from build123d import *

# Parameters (mm, degrees)
SKETCH1_R           = 11.8
SKETCH1_R_2         = 1.4
BOSS_EXTRUDE2_DEPTH = 10


with BuildPart() as part:
    # Sketch1 → Boss-Extrude2 (new body)
    with BuildSketch(Plane(origin=(0, 0, 0), x_dir=(1, 0, 0), z_dir=(0, 1, 0))):
        Polygon((-12.5, 10.5), (-10.5, 12.5), (10.5, 12.5), (12.5, 10.5), (12.5, -10.5), (10.5, -12.5), (-10.5, -12.5), (-12.5, -10.5), align=None)
        with Locations(Location((0, 0, 0), (0, 0, 270))):
            Circle(SKETCH1_R, mode=Mode.SUBTRACT)
        with Locations(Location((-10, 10, 0), (0, 0, 270))):
            Circle(SKETCH1_R_2, mode=Mode.SUBTRACT)
        with Locations(Location((10, 10, 0), (0, 0, 270))):
            Circle(SKETCH1_R_2, mode=Mode.SUBTRACT)
        with Locations(Location((10, -10, 0), (0, 0, 270))):
            Circle(SKETCH1_R_2, mode=Mode.SUBTRACT)
        with Locations(Location((-10, -10, 0), (0, 0, 270))):
            Circle(SKETCH1_R_2, mode=Mode.SUBTRACT)
    extrude(amount=BOSS_EXTRUDE2_DEPTH)


solid = part.part
Can you work these out from the model? Positions are in its coordinate system, mm. Coordinates: 2 decimals unless noted, no trailing zeros. Write each loop counter-clockwise with the first axis right and the second up, starting at its lowest first coordinate (ties: lowest second). Pieces come first, ordered by that corner, then holes. Notation, with made-up numbers: (83, 25) -> (123, 25) arc R20 cw to (123, 42) -> close; hole circle Ø10 at (73.5, -16.5). An arc over 180 degrees is marked (long way). Write each question's results on one line, items separated by ' | '. Start each with the question number.
Q1. We'd pull the mould along X, two halves only. Please class faces 1 (the face through (10.95, 4.93, 8.97)), 2 (the face through (-12.5, 5, 0)), 3 (the face through (12, 5, 11)), 4 (the face through (10.95, 4.93, -11.03)): +X half, -X half, draft (parallel to the pull), parting line (faces both ways), or undercut.
Q2. Imagine slicing it at B-B (z = 0). Write out the boundary of the cut face in (x, y).
Q3. If I drill on probe 1 along X at (y, z) = (7.25, -10); probe 2 along Z at (x, y) = (10.75, 0.75); probe 3 along X at (y, z) = (6, -9), over which ranges is the centre line in solid material (lowest first)?
Q4. I'm going to push a flat-ended pin straight in: pin 1 (2.5 mm diameter, centred on x = 10, z = -10, fed in from -Y). Where does the tip first touch, or does it pass through?
Q5. Imagine slicing it at D-D (x = 10). Write out the boundary of the cut face in (y, z).
Q6. Imagine slicing it at C-C (y = 3.75). Write out the boundary of the cut face in (x, z).
Q7. Imagine slicing it at A-A (x = 0). Write out the boundary of the cut face in (y, z), then the cut area to 3 significant figures.
Taken from the geometry:
1) face 1: undercut | face 2: -X half | face 3: +X half | face 4: undercut
2) outline: (-12.5, 0) -> (-11.8, 0) -> (-11.8, 10) -> (-12.5, 10) -> close; (11.8, 0) -> (12.5, 0) -> (12.5, 10) -> (11.8, 10) -> close
3) probe 1: x = -12.5 to -11.4, -8.6 to -6.26, 6.26 to 8.6, 11.4 to 12.5 | probe 2: z = -12.25 to -11.18, -8.82 to -4.87, 4.87 to 8.82, 11.18 to 12.25 | probe 3: x = -12.5 to -10.98, -9.02 to -7.63, 7.63 to 9.02, 10.98 to 12.5
4) pin 1: passes through
5) outline: (0, -12.5) -> (10, -12.5) -> (10, -11.4) -> (0, -11.4) -> close; (0, -8.6) -> (10, -8.6) -> (10, -6.26) -> (0, -6.26) -> close; (0, 6.26) -> (10, 6.26) -> (10, 8.6) -> (0, 8.6) -> close; (0, 11.4) -> (10, 11.4) -> (10, 12.5) -> (0, 12.5) -> close
6) outline: (-12.5, -10.5) -> (-10.5, -12.5) -> (10.5, -12.5) -> (12.5, -10.5) -> (12.5, 10.5) -> (10.5, 12.5) -> (-10.5, 12.5) -> (-12.5, 10.5) -> close; hole circle Ø23.6 at (0, 0); hole circle Ø2.8 at (-10, -10); hole circle Ø2.8 at (-10, 10); hole circle Ø2.8 at (10, -10); hole circle Ø2.8 at (10, 10)
7) outline: (0, -12.5) -> (10, -12.5) -> (10, -11.8) -> (0, -11.8) -> close; (0, 11.8) -> (10, 11.8) -> (10, 12.5) -> (0, 12.5) -> close | area: 14.0 mm^2
